Could you check a few things on this model? Use its own coordinates, in mm. Face numbers are marked on the shaded views. A direction names the side the tool comes from. Give positions to 0.01 mm unless a question says otherwise; leave off trailing zeros. Order: outer loops, then holes, each group sorted by start corner. A loop starts at its lowest first (then second) coordinate and runs counter-clockwise, first axis right, second up. Notation, with made-up numbers: (-10.5, 66) -> (4.5, 66) arc R24 cw to (4.5, 88) -> close; hole circle Ø11 at (4.25, -20.5). An arc over 180 degrees is marked (long way). Write each question's results on one line, items separated by ' | '.
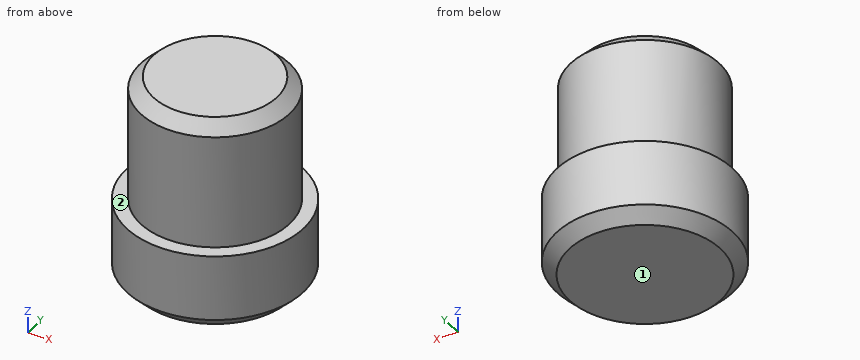
```python
from build123d import *

# Parameters (mm, degrees)
SKETCH_1_R      = 3.5
EXTRUDE_1_DEPTH = 3.1
SKETCH_2_R      = 2.95
EXTRUDE_2_DEPTH = 5
CHAMFER_1_SIZE  = 0.5


with BuildPart() as part:
    # 草图1 → 拉伸1 (new body)
    with BuildSketch(Plane.XY):
        with Locations(Location((0, 0, 0), (0, 0, 180))):
            Circle(SKETCH_1_R)
    extrude(amount=EXTRUDE_1_DEPTH)

    # 草图2 → 拉伸2 (add)
    with BuildSketch(Plane.XY.offset(3.1)):
        Circle(SKETCH_2_R)
    extrude(amount=EXTRUDE_2_DEPTH)

    # 倒角1
    chamfer_1_edges = [part.edges().sort_by_distance(p)[0] for p in [
        (3.5, 0, 0),
        (-2.95, 0, 8.1),
    ]]
    chamfer(chamfer_1_edges, length=CHAMFER_1_SIZE)


solid = part.part
```
Q1. Suppose I cut it at D-D on z = 1. Please give me the cut outline in (x, y), and give its area (3 significant figures).
Here are the results:
outline: circle Ø7 at (0, 0) | area: 38.5 mm²
Q2. I'm going to push flat-ended pins straight in: pin 1 Ø2 at (y, z) = (-2, 1) entering from -X; pin 2 Ø1 at (y, z) = (0, 5.5) entering from -X; pin 3 Ø4 at (x, z) = (-1.5, 6.5) entering from -Y. Where does each tip first touch, or does it pass through?
Here are the results:
pin 1: stops at x = -3.35 | pin 2: stops at x = -2.95 | pin 3: stops at y = -2.95
Q3. Suppose I cut it at A-A on y = 0. Please give me the cut outline in (x, z).
Here are the results:
outline: (-3.5, 0.5) -> (-3, 0) -> (3, 0) -> (3.5, 0.5) -> (3.5, 3.1) -> (2.95, 3.1) -> (2.95, 7.6) -> (2.45, 8.1) -> (-2.45, 8.1) -> (-2.95, 7.6) -> (-2.95, 3.1) -> (-3.5, 3.1) -> close
Q4. Suppose I cut it at C-C on z = 6.5. Please give me the cut outline in (x, y), and give its area (3 significant figures).
Here are the results:
outline: circle Ø5.9 at (0, 0) | area: 27.3 mm²
Q5. For the marked faces 1 and 2, which set-ups out of +Z, -Z, +X, -X, +Y, -Y let a thin tool reach every point of the face, with its end or its side?
Here are the results:
face 1: -Z, +X, -X, +Y, -Y | face 2: +Z
Q6. I need wall thicknesses on line 1 along X through (y, z) = (2.5, 1.5); line 2 along Y through (x, z) = (0, 4); line 3 along Z through (x, y) = (-2.5, -2). Which ranges of each line are inside material? Lowest first, please.
Here are the results:
line 1: x = -2.45 to 2.45 | line 2: y = -2.95 to 2.95 | line 3: z = 0.2 to 3.1
